```python
from build123d import *

# Parameters (mm, degrees)
ESQUISSE1_W      = 28
ESQUISSE1_H      = 10
EXTRUSION1_DEPTH = 10
ESQUISSE2_R      = 4
EXTRUSION2_DEPTH = 32.368774283
ESQUISSE3_R      = 3
EXTRUSION3_DEPTH = 32.368774283


with BuildPart() as part:
    # Esquisse1 → Extrusion1 (new body)
    with BuildSketch(Plane(origin=(0, 0, 0), x_dir=(1, 0, 0), z_dir=(0, 1, 0))):
        with Locations((14, 5)):
            Rectangle(ESQUISSE1_W, ESQUISSE1_H)
    extrude(amount=EXTRUSION1_DEPTH)

    # Esquisse2 → Extrusion2 (cut, through all)
    with BuildSketch(Plane.XY):
        with Locations((14, 5)):
            Circle(ESQUISSE2_R)
    extrude(amount=-EXTRUSION2_DEPTH, mode=Mode.SUBTRACT)

    # Esquisse3 → Extrusion3 (cut, through all)
    with BuildSketch(Plane(origin=(0, 10, 0), x_dir=(1, 0, 0), z_dir=(0, 1, 0))):
        with Locations(Location((5, 5, 0), (0, 0, 270))):
            Circle(ESQUISSE3_R)
        with Locations(Location((23, 5, 0), (0, 0, 270))):
            Circle(ESQUISSE3_R)
    extrude(amount=-EXTRUSION3_DEPTH, mode=Mode.SUBTRACT)


solid = part.part
```
Build history of the part. All positions in model axes, mm. Give positions to 0.01 mm unless a question says otherwise; leave off trailing zeros. Loops run counter-clockwise (first coordinate to the right, second up) from the corner with the lowest first, then second, coordinate; pieces in that order, holes last.
Item 1: Slice it at D-D, the plane z = -1.25. List the corners of the cut face in (x, y), and give its area (3 significant figures).
Answers follow:
outline: (0, 0) - (28, 0) - (28, 10) - (0, 10) - close; hole circle Ø8 at (14, 5)
area: 230 mm2
Item 2: Drill centre lines: line 1 (Y direction, x = 14, z = -5.75); line 2 (X direction, y = 4.5, z = -4.5); line 3 (X direction, y = 9.75, z = -6). Where is each one in solid material? Low to high.
Answers follow:
line 1: y = 0 to 1, 9 to 10
line 2: x = 0 to 2.04, 7.96 to 10.03, 17.97 to 20.04, 25.96 to 28
line 3: x = 0 to 2.17, 7.83 to 20.17, 25.83 to 28
Item 3: Slice it at A-A, the plane z = -5. List the corners of the cut face in (x, y), and give its area (3 significant figures).
Answers follow:
outline: (0, 0) - (2, 0) - (2, 10) - (0, 10) - close; (8, 0) - (20, 0) - (20, 10) - (8, 10) - close; (26, 0) - (28, 0) - (28, 10) - (26, 10) - close; hole circle Ø8 at (14, 5)
area: 110 mm2
Item 4: Slice it at C-C, the plane y = 8.5. List the corners of the cut face in (x, z).
Answers follow:
outline: (0, -10) - (12.06, -10) - (12.06, 0) - (0, 0) - close; (15.94, -10) - (28, -10) - (28, 0) - (15.94, 0) - close; hole circle Ø6 at (5, -5); hole circle Ø6 at (23, -5)
Item 5: Slice it at B-B, the plane x = 23. List the corners of the cut face in (y, z).
Answers follow:
outline: (0, -10) - (10, -10) - (10, -8) - (0, -8) - close; (0, -2) - (10, -2) - (10, 0) - (0, 0) - close
Item 6: Pull direction Z, two halves, no side cores. Call faces 1 (the face through (10, 5, -5)), 2 (the face through (23.9, 5.07, -2.14)), 3 (the face through (13.8, 0.5, -10)): released by +Z, released by -Z, zero draft, split by the parting line, or undercut.
Answers follow:
face 1: zero draft
face 2: undercut
face 3: released by -Z
